Here's how the part is built. I have some questions about the finished solid (model axes, mm). Coordinates: 2 decimals unless noted, no trailing zeros. Write each loop counter-clockwise with the first axis right and the second up, starting at its lowest first coordinate (ties: lowest second). Pieces come first, ordered by that corner, then holes.
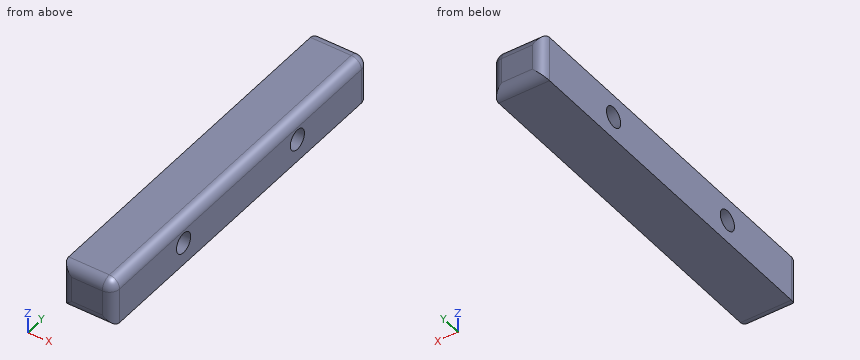
Solid Edge part; units mm, degrees
sketch "Sketch1" plane through (0, 0, 0) normal (0, -1, 0) x (1, 0, 0)
  line L0 (-2.5, -2.25) -> (2.5, -2.25)
  line L1 (2.5, -2.25) -> (2.5, 2.25)
  line L2 (2.5, 2.25) -> (-2.5, 2.25)
  line L3 (-2.5, 2.25) -> (-2.5, -2.25)
  dimension "D1" = 2.5
  dimension "D2" = 2.5
extrude "Protrusion1" add sketch "Sketch1" along normal mid plane 36
fillet "Round_1" radius 1 1 edges at (2.5, 0, 2.25)
hole "Hole_1" at (-2.5, 8, 0) direction (1, 0, 0) diameter 2 end up to next
mirror "Mirror1" about plane through (0, 0, 0) normal (0, -1, 0) of "Hole_1"
fillet "Round_2" radius 1 5 edges at (-0.5, 18, 2.25) (2.2071, 18, 1.9571) (2.5, 18, -0.5) (-2.5, 18, 0) (0, 18, -2.25)
mirror "Mirror2" about plane through (0, 0, 0) normal (0, -1, 0) of "Round_2"
1) Will this pin go through, and if not, where does the flat tip stop? pin 1 (1.2 mm diameter, centred on y = 8, z = 0, fed in from +X).
Values follow:
pin 1: passes through
2) Imagine slicing it at C-C on x = 0.2. Please give me the cut outline in (y, z).
Values follow:
outline: (-18, -1.25) arc R1 ccw to (-17, -2.25) - (17, -2.25) arc R1 ccw to (18, -1.25) - (18, 1.25) arc R1 ccw to (17, 2.25) - (-17, 2.25) arc R1 ccw to (-18, 1.25) - close; hole circle Ø2 at (-8, 0); hole circle Ø2 at (8, 0)
3) Imagine slicing it at B-B on z = 0. Please give me the cut outline in (x, y), then the cut area to 3 significant figures.
Values follow:
outline: (-2.5, -17) arc R1 ccw to (-1.5, -18) - (1.5, -18) arc R1 ccw to (2.5, -17) - (2.5, -9) - (-2.5, -9) - close; (-2.5, -7) - (2.5, -7) - (2.5, 7) - (-2.5, 7) - close; (-2.5, 9) - (2.5, 9) - (2.5, 17) arc R1 ccw to (1.5, 18) - (-1.5, 18) arc R1 ccw to (-2.5, 17) - close
area: 159 mm2
4) Imagine slicing it at D-D on x = 2.2. Please give me the cut outline in (y, z).
Values follow:
outline: (-17.71, -1.95) arc R1 ccw to (-17, -2.25) - (17, -2.25) arc R1 ccw to (17.71, -1.95) - (17.71, 1.25) arc R0.71 ccw to (17, 1.96) - (-17, 1.96) arc R0.71 ccw to (-17.71, 1.25) - close; hole circle Ø2 at (-8, 0); hole circle Ø2 at (8, 0)
5) Imagine slicing it at A-A on y = -8. Please give me the cut outline in (x, z), then the cut area to 3 significant figures.
Values follow:
outline: (-2.5, -2.25) - (2.5, -2.25) - (2.5, -1) - (-2.5, -1) - close; (-2.5, 1) - (2.5, 1) - (2.5, 1.25) arc R1 ccw to (1.5, 2.25) - (-2.5, 2.25) - close
area: 12.3 mm2
6) I need wall thicknesses on probe 1 along Y at (x, z) = (-0.4, 0); probe 2 along Z at (x, y) = (-0.3, 8); probe 3 along Y at (x, z) = (0.85, 1.3). Which ranges of each line are inside material? Lowest first, please.
Values follow:
probe 1: y = -18 to -9, -7 to 7, 9 to 18
probe 2: z = -2.25 to -1, 1 to 2.25
probe 3: y = -18 to 18
